from build123d import *

# Parameters (mm, degrees)
F0_W     = 25.4
F0_H     = 25.4
F0_W_2   = 22.225
F0_H_2   = 22.225
F1_DEPTH = 101.6
F2_R     = 1.5875
F3_DEPTH = 25.4
F4_R     = 1.5875
F5_DEPTH = 25.4


with BuildPart() as f1:
    # F0 (on Front) → F1 (new body)
    with BuildSketch(Plane.XZ):
        Rectangle(F0_W, F0_H)
        Rectangle(F0_W_2, F0_H_2, mode=Mode.SUBTRACT)
    extrude(amount=F1_DEPTH)

    # F2 (on face) → F3 (cut)
    with BuildSketch(Plane.XY.offset(12.7)):
        with Locations((0, -6.35)):
            Circle(F2_R)
        with Locations((0, -19.05)):
            Circle(F2_R)
        with Locations((0, -31.75)):
            Circle(F2_R)
        with Locations((0, -44.45)):
            Circle(F2_R)
        with Locations((0, -57.15)):
            Circle(F2_R)
        with Locations((0, -69.85)):
            Circle(F2_R)
        with Locations((0, -82.55)):
            Circle(F2_R)
        with Locations((0, -95.25)):
            Circle(F2_R)
    extrude(amount=-F3_DEPTH, mode=Mode.SUBTRACT)

    # F4 (on face) → F5 (cut)
    with BuildSketch(Plane.YZ.offset(12.7)):
        with Locations((-6.35, 0)):
            Circle(F4_R)
        with Locations((-19.05, 0)):
            Circle(F4_R)
        with Locations((-31.75, 0)):
            Circle(F4_R)
        with Locations((-44.45, 0)):
            Circle(F4_R)
        with Locations((-57.15, 0)):
            Circle(F4_R)
        with Locations((-69.85, 0)):
            Circle(F4_R)
        with Locations((-82.55, 0)):
            Circle(F4_R)
        with Locations((-95.25, 0)):
            Circle(F4_R)
    extrude(amount=-F5_DEPTH, mode=Mode.SUBTRACT)


solid = f1.part
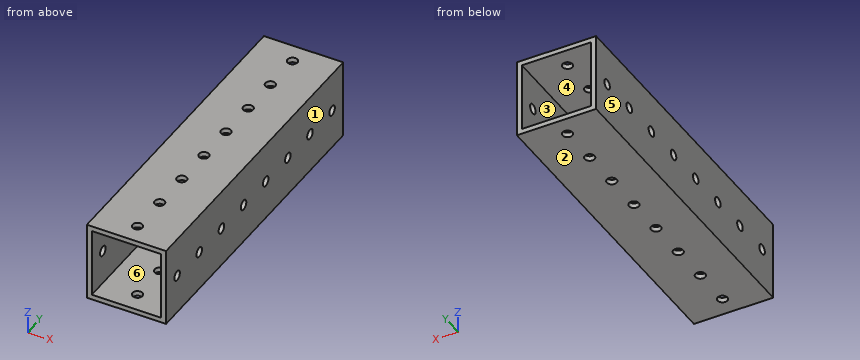
Source: CAD feature listing. Evaluate the final solid. Frame: model axes, mm. Face numbers are marked on the shaded views. A direction names the side the tool comes from. Round coordinates to 2 decimals unless told otherwise and drop trailing zeros. Loops run counter-clockwise (first coordinate to the right, second up) from the corner with the lowest first, then second, coordinate; pieces in that order, holes last. Notation, with made-up numbers: M 63,34 L 112,34 A32 cw 112,62 Z; hole C 2,64 d1. An arc over 180 degrees is marked long. Answer as CSV lines item,"result".
Q1. Reachability of the marked faces 5 and 6 from +Z, -Z, +X, -X, +Y, -Y: full face, straight path, thin tool, end or side. Return the list, or none.
Verdict:
face 5,"+Z, -Z, -X, +Y, -Y"
face 6,"+Y, -Y"
Q2. Cut plane D-D (y = -41.5). Return the cut outline in (x, z), plus the area to 3 significant figures.
Verdict:
outline,"M -12.7,-12.7 L 12.7,-12.7 L 12.7,12.7 L -12.7,12.7 Z; hole M -11.11,-11.11 L 11.11,-11.11 L 11.11,11.11 L -11.11,11.11 Z"
area,"151 mm^2"
Q3. Cut plane B-B (x = -4). Return the cut outline in (y, z), plus the area to 3 significant figures.
Verdict:
outline,"M -101.6,-12.7 L 0,-12.7 L 0,-11.11 L -101.6,-11.11 Z; M -101.6,11.11 L 0,11.11 L 0,12.7 L -101.6,12.7 Z"
area,"323 mm^2"
Q4. Cut plane A-A (y = -6.35). Return the cut outline in (x, z).
Verdict:
outline,"M -12.7,-12.7 L -1.59,-12.7 L -1.59,-11.11 L -11.11,-11.11 L -11.11,-1.59 L -12.7,-1.59 Z; M -12.7,1.59 L -11.11,1.59 L -11.11,11.11 L -1.59,11.11 L -1.59,12.7 L -12.7,12.7 Z; M 1.59,-12.7 L 12.7,-12.7 L 12.7,-1.59 L 11.11,-1.59 L 11.11,-11.11 L 1.59,-11.11 Z; M 1.59,11.11 L 11.11,11.11 L 11.11,1.59 L 12.7,1.59 L 12.7,12.7 L 1.59,12.7 Z"
Q5. Pull-direction query (Z, two-part tool) for the marked faces 1, 2, 3 and 4; classes: +Z half, -Z half, draft (parallel to the pull), parting line (faces both ways), or undercut.
Verdict:
face 1,"draft"
face 2,"-Z half"
face 3,"undercut"
face 4,"undercut"
Q6. Line query: line 1 along Z through (x, y) = (-10.5, -36.5); line 2 along Z through (x, y) = (11.95, -82.55). Output: solid intervals per line, ascending.
Verdict:
line 1,"z = -12.7 to -11.11, 11.11 to 12.7"
line 2,"z = -12.7 to -1.59, 1.59 to 12.7"
Q7. Cut plane C-C (z = 4.25). Return the cut outline in (x, y).
Verdict:
outline,"M -12.7,-101.6 L -11.11,-101.6 L -11.11,0 L -12.7,0 Z; M 11.11,-101.6 L 12.7,-101.6 L 12.7,0 L 11.11,0 Z"
Q8. Contact query for flat-ended pins moving along their axis: pin 1 (3.5 mm diameter, centred on y = -19.05, z = 0, fed in from +X); pin 2 (3 mm diameter, centred on x = 0, y = -69.85, fed in from -Z). Output: stop coordinate, or through.
Verdict:
pin 1,"stops at x = 12.7"
pin 2,"passes through"
